Geometry: final body of the model. Coordinates: model frame, mm. A direction names the side the tool comes from. Give positions to 0.01 mm unless a question says otherwise; leave off trailing zeros. Write each loop counter-clockwise with the first axis right and the second up, starting at its lowest first coordinate (ties: lowest second). Pieces come first, ordered by that corner, then holes.
Q1. Section A-A (y = 0). Return the cut outline in (x, z).
Q2. Section C-C (y = -46.5). Return the cut outline in (x, z).
Q3. Reachability of faces 1 (the flat face through (-67, 0, 15)), 2 (the flat face through (0, -63, 16)) from +Z, -Z, +X, -X, +Y, -Y: full face, straight path, thin tool, end or side. Return the list, or none.
Q4. Mould query, pull axis X, two halves, no side actions, for faces 3 (the flat face through (67, 0, 15)), 4 (the cylindrical face through (-1.71, -73.98, 14.99)), 5 (the cylindrical face through (69.735, 0.806, 14.493)). Classes: +X half, -X half, draft (parallel to the pull), parting line (faces both ways), or undercut.
Q5. Section D-D (z = 14.55). Return the cut outline in (x, y).
Q6. Line query: line 1 (X direction, y = 0, z = 14.8); line 2 (Y direction, x = 0, z = 15.5); line 3 (X direction, y = -51, z = 15.85). Output: solid intervals per line, ascending.
Q7. Section B-B (x = 0). Return the cut outline in (y, z), plus the area to 3 significant figures.
Q8. Pin query (flat end, axial travel): pin 1 Ø1.8 at (x, y) = (-71, 0) entering from -Z; pin 2 Ø4 at (x, y) = (50.2, -50.2) entering from +Z; pin 3 Ø6 at (x, y) = (68, 2.5) entering from +Z; pin 4 Ø1 at (y, z) = (-7, 14.5) entering from -X. Return the tip coordinate at first contact, or that it passes through.
from build123d import *

# Parameters (mm, degrees)
BOX002_W                    = 180
BOX002_H                    = 180
BOX002_DEPTH                = 2
BOX003_W                    = 180
BOX003_H                    = 180
BOX003_DEPTH                = 1
CYLINDER505_R               = 1.5
CYLINDER505_DEPTH           = 60
CYLINDER505_PLACEMENT_ANGLE = 45
CYLINDER504_R               = 1.5
CYLINDER504_DEPTH           = 60
CYLINDER507_R               = 1.5
CYLINDER507_DEPTH           = 60
CYLINDER507_PLACEMENT_ANGLE = 135
CYLINDER506_R               = 1.5
CYLINDER506_DEPTH           = 60
CYLINDER506_PLACEMENT_ANGLE = 225
CYLINDER502_R               = 1.5
CYLINDER502_DEPTH           = 60
CYLINDER501_R               = 1.5
CYLINDER501_DEPTH           = 60
CYLINDER501_PLACEMENT_ANGLE = 45
CYLINDER503_R               = 1.5
CYLINDER503_DEPTH           = 60
TUBE030_R                   = 74
TUBE030_R_2                 = 61
TUBE030_DEPTH               = 2


with BuildPart() as krychle002:
    # Box002 → Box002 (new body)
    with BuildSketch(Plane(origin=(-90, -186, 14), x_dir=(1, 0, 0), z_dir=(0, 0, 1))):
        with Locations((90, 90)):
            Rectangle(BOX002_W, BOX002_H)
    extrude(amount=BOX002_DEPTH)


with BuildPart() as fusion:
    # Box003 → Box003 (new body)
    with BuildSketch(Plane(origin=(-90, -174, 14), x_dir=(1, 0, 0), z_dir=(0, 0, 1))):
        with Locations((90, 90)):
            Rectangle(BOX003_W, BOX003_H)
    extrude(amount=BOX003_DEPTH)

    # Fusion: union Krychle002
    add(krychle002.part)


with BuildPart() as obj1:
    # Cylinder505 → Cylinder505 (new body)
    with BuildSketch(Plane.XY):
        Circle(CYLINDER505_R)
    extrude(amount=CYLINDER505_DEPTH)


with BuildPart() as obj1_1:
    # Cylinder505 placement: moved
    add(obj1.part.moved(Location((50.204581, -50.204581, 0))).rotate(Axis((50.204581, -50.204581, 0), (0, 0, 1)), CYLINDER505_PLACEMENT_ANGLE))


with BuildPart() as obj2:
    # Cylinder504 → Cylinder504 (new body)
    with BuildSketch(Plane(origin=(71, 0, 0), x_dir=(0, 1, 0), z_dir=(0, 0, 1))):
        Circle(CYLINDER504_R)
    extrude(amount=CYLINDER504_DEPTH)


with BuildPart() as obj3:
    # Cylinder507 → Cylinder507 (new body)
    with BuildSketch(Plane.XY):
        Circle(CYLINDER507_R)
    extrude(amount=CYLINDER507_DEPTH)


with BuildPart() as obj3_1:
    # Cylinder507 placement: moved
    add(obj3.part.moved(Location((50.204581, 50.204581, 0))).rotate(Axis((50.204581, 50.204581, 0), (0, 0, 1)), CYLINDER507_PLACEMENT_ANGLE))


with BuildPart() as obj4:
    # Cylinder506 → Cylinder506 (new body)
    with BuildSketch(Plane.XY):
        Circle(CYLINDER506_R)
    extrude(amount=CYLINDER506_DEPTH)


with BuildPart() as obj4_1:
    # Cylinder506 placement: moved
    add(obj4.part.moved(Location((-50.204581, 50.204581, 0))).rotate(Axis((-50.204581, 50.204581, 0), (0, 0, 1)), CYLINDER506_PLACEMENT_ANGLE))


with BuildPart() as obj5:
    # Cylinder502 → Cylinder502 (new body)
    with BuildSketch(Plane(origin=(-71, 0, 0), x_dir=(0, -1, 0), z_dir=(0, 0, 1))):
        Circle(CYLINDER502_R)
    extrude(amount=CYLINDER502_DEPTH)


with BuildPart() as obj6:
    # Cylinder501 → Cylinder501 (new body)
    with BuildSketch(Plane.XY):
        Circle(CYLINDER501_R)
    extrude(amount=CYLINDER501_DEPTH)


with BuildPart() as obj6_1:
    # Cylinder501 placement: moved
    add(obj6.part.moved(Location((-50.204581, -50.204581, 0))).rotate(Axis((-50.204581, -50.204581, 0), (0, 0, -1)), CYLINDER501_PLACEMENT_ANGLE))


with BuildPart() as compound331:
    # Cylinder503 → Cylinder503 (new body)
    with BuildSketch(Plane(origin=(0, -71, 0), x_dir=(1, 0, 0), z_dir=(0, 0, 1))):
        Circle(CYLINDER503_R)
    extrude(amount=CYLINDER503_DEPTH)

    # Compound331: union obj1, obj2, obj3, obj4, obj5, obj6
    add(obj1_1.part)
    add(obj2.part)
    add(obj3_1.part)
    add(obj4_1.part)
    add(obj5.part)
    add(obj6_1.part)


with BuildPart() as obj7:
    # Tube030 → Tube030 (new body)
    with BuildSketch(Plane.XY.offset(14)):
        Circle(TUBE030_R)
        Circle(TUBE030_R_2, mode=Mode.SUBTRACT)
    extrude(amount=TUBE030_DEPTH)

    # Cut205: cut Compound331
    add(compound331.part, mode=Mode.SUBTRACT)

    # Common: intersect Fusion
    add(fusion.part, mode=Mode.INTERSECT)


solid = obj7.part
Computed:
1. outline: (-74, 14) - (-72.5, 14) - (-72.5, 15) - (-74, 15) - close; (-69.5, 14) - (-61, 14) - (-61, 15) - (-69.5, 15) - close; (61, 14) - (69.5, 14) - (69.5, 15) - (61, 15) - close; (72.5, 14) - (74, 14) - (74, 15) - (72.5, 15) - close
2. outline: (-57.57, 14) - (-39.48, 14) - (-39.48, 16) - (-57.57, 16) - close; (39.48, 14) - (57.57, 14) - (57.57, 16) - (39.48, 16) - close
3. face 1: +Z, +X, -X, +Y
3. face 2: +Z, +X, -X, +Y, -Y
4. face 3: draft
4. face 4: parting line
4. face 5: undercut
5. outline: (-73.76, 6) arc R74 ccw (long way) to (73.76, 6) - (60.7, 6) arc R61 cw (long way) to (-60.7, 6) - close; hole circle Ø3 at (-71, 0); hole circle Ø3 at (-50.2, -50.2); hole circle Ø3 at (0, -71); hole circle Ø3 at (50.2, -50.2); hole circle Ø3 at (71, 0)
6. line 1: x = -74 to -72.5, -69.5 to -61, 61 to 69.5, 72.5 to 74
6. line 2: y = -74 to -72.5, -69.5 to -61
6. line 3: x = -53.62 to -51.48, -48.93 to -33.47, 33.47 to 48.93, 51.48 to 53.62
7. outline: (-74, 14) - (-72.5, 14) - (-72.5, 16) - (-74, 16) - close; (-69.5, 14) - (-61, 14) - (-61, 16) - (-69.5, 16) - close
7. area: 20.0 mm2
8. pin 1: passes through
8. pin 2: stops at z = 16
8. pin 3: stops at z = 15
8. pin 4: stops at x = -73.71
